```python
from build123d import *

# Parameters (mm, degrees)
SKETCH1_R           = 3.175
BOSS_EXTRUDE1_DEPTH = 6.35


with BuildPart() as part:
    # Sketch1 → Boss-Extrude1 (new body)
    with BuildSketch(Plane(origin=(0, 0, 0), x_dir=(1, 0, 0), z_dir=(0, 1, 0))):
        with BuildLine():
            ThreePointArc((12.7, 14.199031657), (19.05, 0), (12.7, -14.199031657))
            Line((12.7, -14.199031657), (12.7, -100.803124952))
            ThreePointArc((12.7, -100.803124952), (-4.407318933, -101.504362171), (-21.389473684, -99.322960163))
            Line((-21.389473684, -99.322960163), (-12.7, -58.973007597))
            Line((-12.7, -58.973007597), (-12.7, -14.199031657))
            ThreePointArc((-12.7, -14.199031657), (-19.05, 0), (-12.7, 14.199031657))
            Line((-12.7, 14.199031657), (-12.7, 100.803124952))
            ThreePointArc((-12.7, 100.803124952), (4.407318933, 101.504362171), (21.389473684, 99.322960163))
            Line((21.389473684, 99.322960163), (12.7, 58.973007597))
            Line((12.7, 58.973007597), (12.7, 14.199031657))
        make_face()
        with Locations(Location((0, 0, 0), (0, 0, 270))):
            Circle(SKETCH1_R, mode=Mode.SUBTRACT)
    extrude(amount=BOSS_EXTRUDE1_DEPTH)


solid = part.part
```
Work out the finished part from the listing and answer in its coordinate system (mm). A direction names the side the tool comes from. Coordinates: 2 decimals unless noted, no trailing zeros. Write each loop counter-clockwise with the first axis right and the second up, starting at its lowest first coordinate (ties: lowest second). Pieces come first, ordered by that corner, then holes.
Q1. A cutting plane is placed at B-B, the plane z = 0. Give the vertices of the cut face in (x, y) (3 decimals), then the cut area to 3 significant figures.
Q2. Each of these flat-tipped pins is pushed along its axis until it touches: pin 1 Ø5 at (x, z) = (0.5, 64.5) entering from -Y; pin 2 Ø3 at (y, z) = (3, 29) entering from -X; pin 3 Ø1.9 at (y, z) = (4, 68.5) entering from +X. Where does it stop, or does it pass through?
Q3. Find the intervals of material crossed by line 1 (X direction, y = 2, z = 0) (3 decimals); line 2 (X direction, y = 1, z = -15); line 3 (Z direction, x = 2.5, y = 2), in increasing order.
Q4. A cutting plane is placed at A-A, the plane y = 3.5. Give the vertices of the cut face in (x, z) (3 decimals).
Q5. Which of the six approach directions +Z, -Z, +X, -X, +Y, -Y give full straight-line access (tool end or side, diameter ignored) to faces 4 (the face through (-12.7, 3, -57)), 5 (the face through (17.1, 3.1, -79.4)), 6 (the face through (12.7, 3, 57))?
Q6. A cutting plane is placed at D-D, the plane z = 55.5. Give the vertices of the cut face in (x, y).
Q7. A cutting plane is placed at C-C, the plane x = 0. Give the vertices of the cut face in (y, z) (3 decimals).
Q8. Determine the mould class of faces 1 (the face through (-4.168, 3.131, 101.514)), 2 (the face through (-4, 0, -1)), 3 (the face through (-12.7, 3, 37)) for opening direction Z: released by +Z, released by -Z, zero draft, split by the parting line, or undercut.
Findings below:
1. outline: (-19.05, 0) - (-3.175, 0) - (-3.175, 6.35) - (-19.05, 6.35) - close; (3.175, 0) - (19.05, 0) - (19.05, 6.35) - (3.175, 6.35) - close
1. area: 202 mm2
2. pin 1: stops at y = 0
2. pin 2: stops at x = -12.7
2. pin 3: stops at x = 12.7
3. line 1: x = -19.05 to -3.175, 3.175 to 19.05
3. line 2: x = -12.7 to 12.7
3. line 3: z = -101.57 to -1.96, 1.96 to 101.57
4. outline: (-21.389, 99.323) - (-12.7, 58.973) - (-12.7, 14.199) arc R19.05 ccw to (-12.7, -14.199) - (-12.7, -100.803) arc R101.6 ccw to (21.389, -99.323) - (12.7, -58.973) - (12.7, -14.199) arc R19.05 ccw to (12.7, 14.199) - (12.7, 100.803) arc R101.6 ccw to start; hole circle Ø6.35 at (0, 0)
5. face 4: -Z, -X, +Y, -Y
5. face 5: +X, +Y, -Y
5. face 6: +Z, +X, +Y, -Y
6. outline: (-12.7, 0) - (12.7, 0) - (12.7, 6.35) - (-12.7, 6.35) - close
7. outline: (0, -101.6) - (6.35, -101.6) - (6.35, -3.175) - (0, -3.175) - close; (0, 3.175) - (6.35, 3.175) - (6.35, 101.6) - (0, 101.6) - close
8. face 1: released by +Z
8. face 2: zero draft
8. face 3: undercut
